from build123d import *

# Parameters (mm, degrees)
SKETCH_1_W                   = 40.499972991
SKETCH_1_H                   = 29.6
EXTRUDE_1_DEPTH              = 7
SKETCH_2_W                   = 2
SKETCH_2_H                   = 20.10000001
CUT_EXTRUDE_1_DEPTH          = 54.161241934
SKETCH_3_W                   = 2
SKETCH_3_H                   = 19.399972981
CUT_EXTRUDE_2_DEPTH          = 54.161241934
CUT_EXTRUDE_3_DEPTH          = 2
CUT_EXTRUDE_4_DEPTH          = 2
HOLE_WIZARD_2_5_2_5_1_D      = 2.5
HOLE_WIZARD_3_4_3_4_1_D      = 3.4
HOLE_WIZARD_3_4_3_4_1_DEPTH  = 8
HOLE_WIZARD_M3_1_D           = 3.4
HOLE_WIZARD_M3_1_DEPTH       = 10
HOLE_WIZARD_M3_1_CBORE_D     = 4.7
HOLE_WIZARD_M3_1_CBORE_DEPTH = 2
HOLE_WIZARD_M3_2_D           = 3.3
HOLE_WIZARD_M3_2_DEPTH       = 5
HOLE_WIZARD_M3_2_CBORE_D     = 6.1
HOLE_WIZARD_M3_2_CBORE_DEPTH = 1
FILLET_1_R                   = 0.5
FILLET_2_R                   = 3
FILLET_3_R                   = 5


with BuildPart() as part:
    # 草图1 → 凸台-拉伸1 (new body)
    with BuildSketch(Plane(origin=(-7, 0, 0), x_dir=(0, -1, 0), z_dir=(-1, 0, 0))):
        with Locations((23.349986486, 61.611428686)):
            Rectangle(SKETCH_1_W, SKETCH_1_H)
    extrude(amount=-EXTRUDE_1_DEPTH)

    # 草图2 → 切除-拉伸1 (cut, through all)
    with BuildSketch(Plane(origin=(0, 0, 46.811428686), x_dir=(-1, 0, 0), z_dir=(0, 0, -1))):
        with Locations((6, -13.149999995)):
            Rectangle(SKETCH_2_W, SKETCH_2_H)
    extrude(amount=-CUT_EXTRUDE_1_DEPTH, mode=Mode.SUBTRACT)

    # 草图3 → 切除-拉伸2 (cut, through all)
    with BuildSketch(Plane(origin=(0, 0, 46.811428686), x_dir=(-1, 0, 0), z_dir=(0, 0, -1))):
        with Locations((6, -33.89998649)):
            Rectangle(SKETCH_3_W, SKETCH_3_H)
    extrude(amount=-CUT_EXTRUDE_2_DEPTH, mode=Mode.SUBTRACT)

    # 草图4 → 切除-拉伸3 (cut)
    with BuildSketch(Plane(origin=(0, 0, 0), x_dir=(0, 0, -1), z_dir=(1, 0, 0))):
        with BuildLine():
            Line((-58.961428686, -3.09999999), (-58.961428686, -5.6))
            ThreePointArc((-58.961428686, -5.6), (-56.611428686, -7.95), (-54.261428686, -5.6))
            Line((-54.261428686, -5.6), (-54.261428686, -3.09999999))
            Line((-54.261428686, -3.09999999), (-58.961428686, -3.09999999))
        make_face()
    extrude(amount=-CUT_EXTRUDE_3_DEPTH, mode=Mode.SUBTRACT)

    # 草图5 → 切除-拉伸4 (cut)
    with BuildSketch(Plane(origin=(0, 0, 0), x_dir=(0, 0, -1), z_dir=(1, 0, 0))):
        with BuildLine():
            Line((-68.961428686, -3.09999999), (-68.961428686, -5.6))
            ThreePointArc((-68.961428686, -5.6), (-66.611428686, -7.95), (-64.261428686, -5.6))
            Line((-64.261428686, -5.6), (-64.261428686, -3.09999999))
            Line((-64.261428686, -3.09999999), (-68.961428686, -3.09999999))
        make_face()
    extrude(amount=-CUT_EXTRUDE_4_DEPTH, mode=Mode.SUBTRACT)

    # 草图6 → 旋转1 (revolve)
    with BuildSketch(Plane(origin=(0, -31.7, 0), x_dir=(1, 0, 0), z_dir=(0, 1, 0))):
        Polygon((-10, -57.111428686), (-10, -61.611428686), (-5, -61.611428686), (-5, -53.861428686), (-9, -53.861428686), (-9, -57.111428686), align=None)
    revolve(axis=Axis((-10, -31.7, 61.611428686), (1, 0, 0)))

    # Ø2.5 (2.5) 直径孔1 (through all)
    with Locations(Plane.ZY.offset(5)):
        with Locations((72.411428686, -5.599972981), (50.811428686, -20.599972981), (72.411428686, -20.599972981), (50.811428686, -5.599972981)):
            Hole(HOLE_WIZARD_2_5_2_5_1_D / 2)

    # Ø3.4 (3.4) 直径孔1
    with Locations(Plane(origin=(-2, 0, 0), x_dir=(0, 0, -1), z_dir=(1, 0, 0))):
        with Locations((-56.611428686, -5.6), (-66.611428686, -5.6)):
            Hole(HOLE_WIZARD_3_4_3_4_1_D / 2, depth=HOLE_WIZARD_3_4_3_4_1_DEPTH)

    # M3 六角头机械螺钉的柱形沉头孔1
    with Locations(Plane(origin=(0, 0, 0), x_dir=(0, 0, -1), z_dir=(1, 0, 0))):
        with Locations((-56.611428686, -20.6), (-66.611428686, -20.6)):
            CounterBoreHole(HOLE_WIZARD_M3_1_D / 2, HOLE_WIZARD_M3_1_CBORE_D / 2, HOLE_WIZARD_M3_1_CBORE_DEPTH, depth=HOLE_WIZARD_M3_1_DEPTH)

    # M3 六角头机械螺钉的柱形沉头孔2
    with Locations(Plane.ZY.offset(10)):
        with Locations((61.611428686, -31.7)):
            CounterBoreHole(HOLE_WIZARD_M3_2_D / 2, HOLE_WIZARD_M3_2_CBORE_D / 2, HOLE_WIZARD_M3_2_CBORE_DEPTH, depth=HOLE_WIZARD_M3_2_DEPTH)

    # 圆角1
    fillet_1_edges = [part.edges().sort_by_distance(p)[0] for p in [
        (-1, -3.09999999, 58.961428686),
        (-1, -3.09999999, 54.261428686),
        (-1, -3.09999999, 68.961428686),
        (-1, -3.09999999, 64.261428686),
    ]]
    fillet(fillet_1_edges, radius=FILLET_1_R)

    # 圆角2
    fillet_2_edges = [part.edges().sort_by_distance(p)[0] for p in [
        (-2.5, -3.09999999, 76.411428686),
        (-2.5, -43.599972981, 76.411428686),
        (-2.5, -43.599972981, 46.811428686),
        (-2.5, -3.09999999, 46.811428686),
    ]]
    fillet(fillet_2_edges, radius=FILLET_2_R)

    # 圆角3
    fillet_3_edges = [part.edges().sort_by_distance(p)[0] for p in [
        (-6, -24.2, 59.658866267),
        (-6, -24.2, 63.563991105),
    ]]
    fillet(fillet_3_edges, radius=FILLET_3_R)


solid = part.part
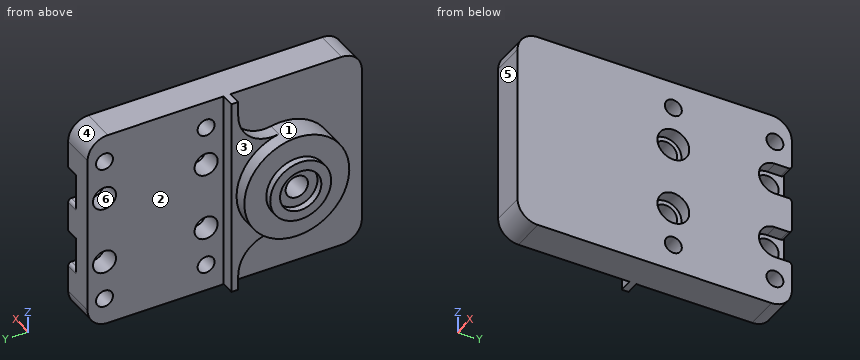
Here's how the part is built. I have some questions about the finished solid (model axes, mm). Face numbers are marked on the shaded views. A direction names the side the tool comes from. Coordinates: 2 decimals unless noted, no trailing zeros. Write each loop counter-clockwise with the first axis right and the second up, starting at its lowest first coordinate (ties: lowest second). Pieces come first, ordered by that corner, then holes.
Item 1: If we mould it in two halves opening along Y, with no side actions, what happens to the marked faces 4, 5 and 6? For each: +Y half, -Y half, draft (parallel to the pull), parting line (faces both ways), or undercut.
Item 2: I want a section at B-B on z = 55.5. Write out the boundary of the cut face in (x, y).
Item 3: If I drill on line 1 (Y direction, x = -3.5, z = 49.75); line 2 (Y direction, x = -3, z = 57.5); line 3 (X direction, y = -5.5, z = 59.5), over which ranges is the centre line in solid material (lowest first)?
Item 4: I want a section at A-A on x = -3.5. Count the separate pieces of the cut face and the enclosed holes in it, and give its area (3 significant figures).
Item 5: I want a section at D-D on x = -9.5. Write out the boundary of the cut face in (y, z).
Item 6: I want a section at C-C on y = -31.7. Write out the boundary of the cut face in (x, z).
Item 7: On a 3-axis mill with a long thin cutter (end or side, diameter ignored), from which of +Z, -Z, +X, -X, +Y, -Y can I reach the whole of each face in a straight line? I mean the marked faces 1, 2 and 3. Say none if no direction works.
Item 8: Will these pins go through, and if not, where does the flat tip stop? pin 1 (1 mm diameter, centred on x = -1, y = -5, fed in from -Z); pin 2 (1.5 mm diameter, centred on y = -6.5, z = 65.5, fed in from +X); pin 3 (2.5 mm diameter, centred on y = -32, z = 61.5, fed in from -X); pin 4 (1.5 mm diameter, centred on y = -20.6, z = 50.81, fed in from -X).
Findings below:
1. face 4: +Y half
1. face 5: -Y half
1. face 6: undercut
2. outline: (-9, -36.47) - (-5, -36.47) - (-5, -43.6) - (0, -43.6) - (0, -22.67) - (-2, -22.67) - (-2, -21.89) - (-5, -21.89) - (-5, -23.2) - (-7, -23.2) - (-7, -26.93) - (-9, -26.93) - close; (-5, -19.31) - (-2, -19.31) - (-2, -18.53) - (0, -18.53) - (0, -7.67) - (-2, -7.67) - (-2, -6.89) - (-5, -6.89) - close; (-5, -4.31) - (-2, -4.31) - (-2, -3.1) - (-5, -3.1) - close
3. line 1: y = -43.6 to -21.26, -19.94 to -6.26, -4.94 to -3.1
3. line 2: y = -43.6 to -22.05, -19.15 to -7.05, -4.15 to -3.1
3. line 3: x = -5 to 0
4. separate pieces: 1
4. enclosed holes: 8
4. area: 1,140 mm2
5. outline: circle Ø9 at (-31.7, 61.61); hole circle Ø6.1 at (-31.7, 61.61)
6. outline: (-10, 57.11) - (-9, 57.11) - (-9, 53.86) - (-5, 53.86) - (-5, 46.81) - (0, 46.81) - (0, 76.41) - (-5, 76.41) - (-5, 69.36) - (-9, 69.36) - (-9, 66.11) - (-10, 66.11) - (-10, 64.66) - (-9, 64.66) - (-9, 63.26) - (-5, 63.26) - (-5, 59.96) - (-9, 59.96) - (-9, 58.56) - (-10, 58.56) - close
7. face 1: -X
7. face 2: +Z, -Z, -X, +Y
7. face 3: -X, +Y
8. pin 1: stops at z = 46.87
8. pin 2: stops at x = -2
8. pin 3: stops at x = -5
8. pin 4: passes through
